from build123d import *

# Parameters (mm, degrees)
BOSS_EXTRUDE1_DEPTH        = 9.525
SKETCH2_W                  = 509.27
SKETCH2_H                  = 35.56
CUT_EXTRUDE1_DEPTH         = 3.175
SKETCH3_R                  = 2.286
CUT_EXTRUDE2_DEPTH         = 595.632661817
F_10_32_TAPPED_HOLE1_D     = 4.0386
F_10_32_TAPPED_HOLE1_DEPTH = 13.716
F_10_32_TAPPED_HOLE1_TIP   = 1.213317848
F_10_32_TAPPED_HOLE2_D     = 4.0386
F_10_32_TAPPED_HOLE2_DEPTH = 13.716
F_10_32_TAPPED_HOLE2_TIP   = 1.213317848
SKETCH8_R                  = 38.1
BOSS_EXTRUDE2_DEPTH        = 6.35
SKETCH9_R                  = 20.447
BOSS_EXTRUDE3_DEPTH        = 5.08
SKETCH10_R                 = 12.573
BOSS_EXTRUDE4_DEPTH        = 19.05
F_10_24_TAPPED_HOLE1_D     = 3.7973
F_10_24_TAPPED_HOLE1_DEPTH = 14.986
F_10_24_TAPPED_HOLE1_TIP   = 1.140824014
FILLET2_R                  = 2.54


with BuildPart() as part:
    # Sketch1 → Boss-Extrude1 (new body)
    with BuildSketch(Plane.XY):
        with BuildLine():
            Line((103.778975516, 188.321024484), (137.521024484, 154.578975516))
            ThreePointArc((137.521024484, 154.578975516), (154.001730604, 143.566919748), (173.442048969, 139.7))
            Line((173.442048969, 139.7), (334.557951031, 139.7))
            ThreePointArc((334.557951031, 139.7), (353.998269396, 143.566919748), (370.478975516, 154.578975516))
            Line((370.478975516, 154.578975516), (404.221024484, 188.321024484))
            ThreePointArc((404.221024484, 188.321024484), (420.701730604, 199.333080252), (440.142048969, 203.2))
            Line((440.142048969, 203.2), (482.6, 203.2))
            ThreePointArc((482.6, 203.2), (536.481536726, 180.881536726), (558.8, 127))
            Line((558.8, 127), (558.8, 76.2))
            ThreePointArc((558.8, 76.2), (536.481536726, 22.318463274), (482.6, 0))
            Line((482.6, 0), (440.142048969, 0))
            ThreePointArc((440.142048969, 0), (420.701730604, 3.866919748), (404.221024484, 14.878975516))
            Line((404.221024484, 14.878975516), (370.478975516, 48.621024484))
            ThreePointArc((370.478975516, 48.621024484), (353.998269396, 59.633080252), (334.557951031, 63.5))
            Line((334.557951031, 63.5), (173.442048969, 63.5))
            ThreePointArc((173.442048969, 63.5), (154.001730604, 59.633080252), (137.521024484, 48.621024484))
            Line((137.521024484, 48.621024484), (103.778975516, 14.878975516))
            ThreePointArc((103.778975516, 14.878975516), (87.298269396, 3.866919748), (67.857951031, 0))
            Line((67.857951031, 0), (0, 0))
            Line((0, 0), (0, 203.2))
            Line((0, 203.2), (67.857951031, 203.2))
            ThreePointArc((67.857951031, 203.2), (87.298269396, 199.333080252), (103.778975516, 188.321024484))
        make_face()
    extrude(amount=BOSS_EXTRUDE1_DEPTH)

    # Sketch2 → Cut-Extrude1 (cut)
    with BuildSketch(Plane.XY.offset(9.525)):
        with Locations((297.815, 101.6)):
            Rectangle(SKETCH2_W, SKETCH2_H)
    extrude(amount=-CUT_EXTRUDE1_DEPTH, mode=Mode.SUBTRACT)

    # Sketch3 → Cut-Extrude2 (cut, through all)
    with BuildSketch(Plane.XY.offset(6.35)):
        with Locations((532.765, 101.6)):
            Circle(SKETCH3_R)
        with Locations((58.039, 101.6)):
            Circle(SKETCH3_R)
        with Locations((509.905, 101.6)):
            Circle(SKETCH3_R)
        with Locations((496.45, 101.6)):
            Circle(SKETCH3_R)
        with Locations((76.44999999, 101.6)):
            Circle(SKETCH3_R)
    extrude(amount=-CUT_EXTRUDE2_DEPTH, mode=Mode.SUBTRACT)

    # #10-32 Tapped Hole1
    with Locations(Plane(origin=(0, 203.2, 0), x_dir=(-1, 0, 0), z_dir=(0, 1, 0))):
        with Locations((-12.7, 4.7625), (-50.8, 4.7625), (-461.01, 4.7625)):
            Hole(F_10_32_TAPPED_HOLE1_D / 2, depth=F_10_32_TAPPED_HOLE1_DEPTH)
            with Locations((0, 0, -(F_10_32_TAPPED_HOLE1_DEPTH + F_10_32_TAPPED_HOLE1_TIP / 2))):  # 118° drill point
                Cone(0, F_10_32_TAPPED_HOLE1_D / 2, F_10_32_TAPPED_HOLE1_TIP, mode=Mode.SUBTRACT)

    # #10-32 Tapped Hole2
    with Locations(Plane.XZ):
        with Locations((12.7, 4.7625), (50.8, 4.7625), (461.01, 4.7625)):
            Hole(F_10_32_TAPPED_HOLE2_D / 2, depth=F_10_32_TAPPED_HOLE2_DEPTH)
            with Locations((0, 0, -(F_10_32_TAPPED_HOLE2_DEPTH + F_10_32_TAPPED_HOLE2_TIP / 2))):  # 118° drill point
                Cone(0, F_10_32_TAPPED_HOLE2_D / 2, F_10_32_TAPPED_HOLE2_TIP, mode=Mode.SUBTRACT)

    # Sketch8 → Boss-Extrude2 (add)
    with BuildSketch(Plane(origin=(0, 0, 0), x_dir=(-1, 0, 0), z_dir=(0, 0, -1))):
        with Locations(Location((-279.4, 101.6, 0), (0, 0, 270))):
            Circle(SKETCH8_R)
    extrude(amount=BOSS_EXTRUDE2_DEPTH)

    # Sketch9 → Boss-Extrude3 (add)
    with BuildSketch(Plane(origin=(0, 0, -6.35), x_dir=(-1, 0, 0), z_dir=(0, 0, -1))):
        with Locations((-279.4, 101.6)):
            Circle(SKETCH9_R)
    extrude(amount=BOSS_EXTRUDE3_DEPTH)

    # Sketch10 → Boss-Extrude4 (add)
    with BuildSketch(Plane(origin=(0, 0, -11.43), x_dir=(-1, 0, 0), z_dir=(0, 0, -1))):
        with Locations(Location((-279.4, 101.6, 0), (0, 0, 180))):
            Circle(SKETCH10_R)
    extrude(amount=BOSS_EXTRUDE4_DEPTH)

    # #10-24 Tapped Hole1
    with Locations(Plane(origin=(0, 0, -30.48), x_dir=(-1, 0, 0), z_dir=(0, 0, -1))):
        with Locations((-279.4, 101.6)):
            Hole(F_10_24_TAPPED_HOLE1_D / 2, depth=F_10_24_TAPPED_HOLE1_DEPTH)
            with Locations((0, 0, -(F_10_24_TAPPED_HOLE1_DEPTH + F_10_24_TAPPED_HOLE1_TIP / 2))):  # 118° drill point
                Cone(0, F_10_24_TAPPED_HOLE1_D / 2, F_10_24_TAPPED_HOLE1_TIP, mode=Mode.SUBTRACT)

    # Fillet2
    fillet2_edges = [part.edges().sort_by_distance(p)[0] for p in [
        (0, 101.6, 0),
    ]]
    fillet(fillet2_edges, radius=FILLET2_R)


solid = part.part
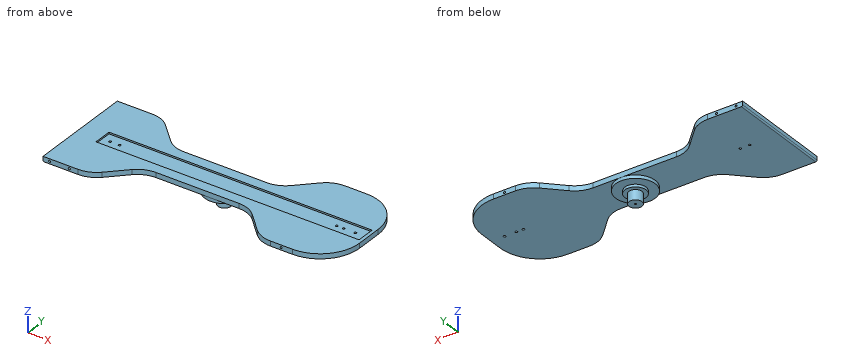
The listing builds one solid part. Answer for the finished solid, in the listing's coordinates (mm). Give positions to 0.01 mm unless a question says otherwise; leave off trailing zeros. Loops run counter-clockwise (first coordinate to the right, second up) from the corner with the lowest first, then second, coordinate; pieces in that order, holes last. Notation, with made-up numbers: (84, -16) - (100, -16) arc R15 ccw to (100, 8) - close; hole circle Ø3 at (48.5, 51.5). An arc over 180 degrees is marked (long way). Answer as a JSON object with one key per item and string values.
1. A cutting plane is placed at B-B (x = 308.5). Write down the section's boundary in (y, z) (3 decimals).
Determined:
{"outline": "(63.5, 0) - (77.007, 0) - (77.007, -6.35) - (126.193, -6.35) - (126.193, 0) - (139.7, 0) - (139.7, 9.525) - (119.38, 9.525) - (119.38, 6.35) - (83.82, 6.35) - (83.82, 9.525) - (63.5, 9.525) - close"}
2. A cutting plane is placed at A-A (y = 173). Write down the section's boundary in (x, z) (3 decimals).
Determined:
{"outline": "(0, 2.54) arc R2.54 ccw to (2.54, 0) - (119.1, 0) - (119.1, 9.525) - (0, 9.525) - close; (388.9, 0) - (543.349, 0) - (543.349, 9.525) - (388.9, 9.525) - close"}
3. Flat-ended cylindrical pins translate along their axes: pin 1 Ø5.5 at (x, y) = (532.765, 101.6) entering from +Z; pin 2 Ø3 at (x, z) = (461.01, 4.76) entering from +Y; pin 3 Ø2.5 at (x, z) = (12.7, 4.76) entering from +Y. Find the tip coordinate at first contact, or state that the pin passes through.
Determined:
{"pin 1": "z = 6.35", "pin 2": "y = 189.17", "pin 3": "y = 189.02"}
4. Find the intervals of material crossed by L1, parallel to X at y = 101, z = 5; L2, parallel to X at y = 101, z = 1; L3, parallel to Z at x = 461.01, y = 3.5 (3 decimals), in increasing order. Write a range as [from, to].
Determined:
{"L1": "[0, 55.83], [60.24, 74.24], [78.66, 494.24], [498.66, 507.7], [512.11, 530.56], [534.97, 558.8]", "L2": "[0.52, 55.83], [60.24, 74.24], [78.66, 494.24], [498.66, 507.7], [512.11, 530.56], [534.97, 558.8]", "L3": "[0, 2.743], [6.782, 9.525]"}
